Verification items for the finished model (mm, model axes). A direction names the side the tool comes from. Round coordinates to 2 decimals unless told otherwise and drop trailing zeros. Write each loop counter-clockwise with the first axis right and the second up, starting at its lowest first coordinate (ties: lowest second). Pieces come first, ordered by that corner, then holes. Notation, with made-up numbers: (14, 87) - (69, 87) arc R9 ccw to (69, 91) - close; hole circle Ø2 at (63.25, 47). An arc over 180 degrees is marked (long way). Answer as a JSON object with one key per item and string values.
```python
from build123d import *

# Parameters (mm, degrees)
PAD002_DEPTH           = 120
SKETCH012_W            = 44
SKETCH012_H            = 120
PAD003_DEPTH           = 2
LINEARPATTERN001_COUNT = 3
LINEARPATTERN001_PITCH = 15
SKETCH013_R            = 3
POCKET_DEPTH           = 5
SKETCH014_R            = 3
POCKET012_DEPTH        = 5
SKETCH016_R            = 4.15
POCKET013_DEPTH        = 1
POCKET013_DEPTH_BACK   = -8
SKETCH017_R            = 4.15
POCKET014_DEPTH        = 1
POCKET014_DEPTH_BACK   = -8
SKETCH_W               = 1.5
SKETCH_H               = 20
PAD_DEPTH              = 0.4


with BuildPart() as part:
    # Sketch011 → Pad002 (new body)
    with BuildSketch(Plane.XZ):
        Polygon((7, -6), (7, 6), (5.1, 6), (5.1, 5), (6.1, 4), (6.1, 3.2), (5.1, 3.2), (5.1, -4), (-5.1, -4), (-5.1, 3.2), (-6.1, 3.2), (-6.1, 4), (-5.1, 5), (-5.1, 6), (-7, 6), (-7, -6), align=None)
    pad002 = extrude(amount=PAD002_DEPTH)

    # Sketch012 (on DatumPlane) → Pad003 (join)
    with BuildSketch(Plane.XY.offset(-6)):
        with Locations((15, -60)):
            Rectangle(SKETCH012_W, SKETCH012_H)
    extrude(amount=PAD003_DEPTH)

    # LinearPattern001: Pad002 ×3
    with Locations(*[(i * LINEARPATTERN001_PITCH, 0, 0) for i in range(1, LINEARPATTERN001_COUNT)]):
        add(pad002)

    # Sketch013 → Pocket (cut)
    with BuildSketch(Plane(origin=(-15, -215.5, -4), x_dir=(1, 0, 0), z_dir=(0, 0, 1))):
        with Locations((15, 95.5)):
            Circle(SKETCH013_R)
        with Locations((45, 95.5)):
            Circle(SKETCH013_R)
        with Locations((30, 110.5)):
            Circle(SKETCH013_R)
        with Locations((15, 125.5)):
            Circle(SKETCH013_R)
        with Locations((45, 125.5)):
            Circle(SKETCH013_R)
        with Locations((15, 155.5)):
            Circle(SKETCH013_R)
        with Locations((45, 155.5)):
            Circle(SKETCH013_R)
        with Locations((30, 140.5)):
            Circle(SKETCH013_R)
        with Locations((30, 170.5)):
            Circle(SKETCH013_R)
        with Locations((15, 185.5)):
            Circle(SKETCH013_R)
        with Locations((45, 185.5)):
            Circle(SKETCH013_R)
        with Locations((30, 200.5)):
            Circle(SKETCH013_R)
        with Locations((15, 215.5)):
            Circle(SKETCH013_R)
        with Locations((45, 215.5)):
            Circle(SKETCH013_R)
    extrude(amount=-POCKET_DEPTH, mode=Mode.SUBTRACT)

    # Sketch014 → Pocket012 (cut)
    with BuildSketch(Plane(origin=(0, -215.5, -4), x_dir=(1, 0, 0), z_dir=(0, 0, 1))):
        with Locations((15, 95.5)):
            Circle(SKETCH014_R)
        with Locations((30, 110.5)):
            Circle(SKETCH014_R)
        with Locations((15, 125.5)):
            Circle(SKETCH014_R)
        with Locations((15, 155.5)):
            Circle(SKETCH014_R)
        with Locations((30, 140.5)):
            Circle(SKETCH014_R)
        with Locations((30, 170.5)):
            Circle(SKETCH014_R)
        with Locations((15, 185.5)):
            Circle(SKETCH014_R)
        with Locations((30, 200.5)):
            Circle(SKETCH014_R)
        with Locations((15, 215.5)):
            Circle(SKETCH014_R)
        with Locations((45, 215.5)):
            Circle(SKETCH014_R)
        with Locations((0, 110.5)):
            Circle(SKETCH014_R)
        with Locations((0, 140.5)):
            Circle(SKETCH014_R)
        with Locations((0, 170.5)):
            Circle(SKETCH014_R)
        with Locations((0, 200.5)):
            Circle(SKETCH014_R)
    extrude(amount=-POCKET012_DEPTH, mode=Mode.SUBTRACT)

    # Sketch016 → Pocket013 (cut, two sides)
    with BuildSketch(Plane(origin=(-15, -215.5, -4), x_dir=(1, 0, 0), z_dir=(0, 0, 1))) as pocket013_sk:
        with Locations((15, 95.5)):
            Circle(SKETCH016_R)
        with Locations((45, 95.5)):
            Circle(SKETCH016_R)
        with Locations((30, 110.5)):
            Circle(SKETCH016_R)
        with Locations((15, 125.5)):
            Circle(SKETCH016_R)
        with Locations((45, 125.5)):
            Circle(SKETCH016_R)
        with Locations((15, 155.5)):
            Circle(SKETCH016_R)
        with Locations((45, 155.5)):
            Circle(SKETCH016_R)
        with Locations((30, 140.5)):
            Circle(SKETCH016_R)
        with Locations((30, 170.5)):
            Circle(SKETCH016_R)
        with Locations((15, 185.5)):
            Circle(SKETCH016_R)
        with Locations((45, 185.5)):
            Circle(SKETCH016_R)
        with Locations((30, 200.5)):
            Circle(SKETCH016_R)
        with Locations((15, 215.5)):
            Circle(SKETCH016_R)
        with Locations((45, 215.5)):
            Circle(SKETCH016_R)
    extrude(amount=-POCKET013_DEPTH, mode=Mode.SUBTRACT)
    extrude(pocket013_sk.sketch, amount=-POCKET013_DEPTH_BACK, mode=Mode.SUBTRACT)

    # Sketch017 → Pocket014 (cut, two sides)
    with BuildSketch(Plane(origin=(0, -215.5, -4), x_dir=(1, 0, 0), z_dir=(0, 0, 1))) as pocket014_sk:
        with Locations((15, 95.5)):
            Circle(SKETCH017_R)
        with Locations((30, 110.5)):
            Circle(SKETCH017_R)
        with Locations((15, 125.5)):
            Circle(SKETCH017_R)
        with Locations((15, 155.5)):
            Circle(SKETCH017_R)
        with Locations((30, 140.5)):
            Circle(SKETCH017_R)
        with Locations((30, 170.5)):
            Circle(SKETCH017_R)
        with Locations((15, 185.5)):
            Circle(SKETCH017_R)
        with Locations((30, 200.5)):
            Circle(SKETCH017_R)
        with Locations((15, 215.5)):
            Circle(SKETCH017_R)
        with Locations((45, 215.5)):
            Circle(SKETCH017_R)
        with Locations((0, 110.5)):
            Circle(SKETCH017_R)
        with Locations((0, 140.5)):
            Circle(SKETCH017_R)
        with Locations((0, 170.5)):
            Circle(SKETCH017_R)
        with Locations((0, 200.5)):
            Circle(SKETCH017_R)
    extrude(amount=-POCKET014_DEPTH, mode=Mode.SUBTRACT)
    extrude(pocket014_sk.sketch, amount=-POCKET014_DEPTH_BACK, mode=Mode.SUBTRACT)

    # Sketch (on Face7 of Pocket014) → Pad (join)
    with BuildSketch(Plane(origin=(-7, 0, 0), x_dir=(0, 0, -1), z_dir=(-1, 0, 0))):
        with Locations((5.25, 110)):
            Rectangle(SKETCH_W, SKETCH_H)
    extrude(amount=PAD_DEPTH)


with BuildPart() as part_1:
    # Body001 placement: moved
    add(part.part.moved(Location((18.5, -36, 9))))


solid = part_1.part
```
1. Cross-section at A-A (z = 8.75). Record the boundary of the cut face in (x, y), plus the area to 3 significant figures.
Completed:
{"outline": "(11.5, -156) - (13.4, -156) - (13.4, -36) - (11.5, -36) - close; (23.6, -156) - (25.5, -156) - (25.5, -36) - (23.6, -36) - close; (26.5, -156) - (28.4, -156) - (28.4, -36) - (26.5, -36) - close; (38.6, -156) - (40.5, -156) - (40.5, -36) - (38.6, -36) - close; (41.5, -156) - (43.4, -156) - (43.4, -36) - (41.5, -36) - close; (53.6, -156) - (55.5, -156) - (55.5, -36) - (53.6, -36) - close", "area": "1,370 mm^2"}
2. Access from +Z, -Z, +X, -X, +Y, -Y to the whole of each face (thin tool, end or side, straight path). Record for faces 1 (the face through (47.5, -39, 4)), 2 (the face through (17.6, -130.05, 4.51)), 3 (the face through (40.5, -95, 10)).
Completed:
{"face 1": "+Z, +Y", "face 2": "+Z", "face 3": "+Z, +Y, -Y"}
3. Mould release check, pull along Y, two halves, no side actions. Record for faces 4 (the face through (35.73, -92.5, 4.51)), 5 (the face through (13.4, -95, 9)), 6 (the face through (33.59, -151.85, 4.51)): released by +Y, released by -Y, zero draft, split by the parting line, or undercut.
Completed:
{"face 4": "undercut", "face 5": "zero draft", "face 6": "released by -Y"}
4. Go/stop test with flat-tipped pins: pin 1 (4 mm diameter, centred on x = 35, y = -127, fed in from +Z); pin 2 (3 mm diameter, centred on y = -93, z = 12.5, fed in from -X); pin 3 (9.5 mm diameter, centred on x = 18.5, y = -81, fed in from -Z); pin 4 (1 mm diameter, centred on x = 23, z = 6.5, fed in from -Y). Record where each tip stops, or that it passes through.
Completed:
{"pin 1": "stops at z = 4", "pin 2": "stops at x = 11.5", "pin 3": "stops at z = 3", "pin 4": "passes through"}
5. Cross-section at B-B (y = -141). Count the separate pieces of the cut face and the enclosed holes in it, plus the area to 3 significant figures.
Completed:
{"separate pieces": "4", "enclosed holes": "0", "area": "152 mm^2"}
6. Material ranges on probe 1 along X at (y, z) = (-70.5, 5.25); probe 2 along X at (y, z) = (-69.5, 13); probe 3 along X at (y, z) = (-48.5, 4.5), recorded low to high. Write a range as from..to.
Completed:
{"probe 1": "x = 11.5..13.4, 23.6..25.5, 26.5..28.4, 38.6..40.5, 41.5..43.4, 53.6..55.5", "probe 2": "x = 11.5..12.4, 24.6..25.5, 26.5..27.4, 39.6..40.5, 41.5..42.4, 54.6..55.5", "probe 3": "x = 11.5..15.19, 21.81..30.19, 36.81..45.19, 51.81..55.5"}
